from build123d import *

# Parameters (mm, degrees)
MAIN_DEPTH                   = 37.5
SKETCH2_W                    = 41
SKETCH2_H                    = 21
SERVOPLACE_DEPTH             = 11
SKETCH3_R                    = 1.25
SERVOFIXHOLE_DEPTH           = 11
SKETCH4_W                    = 10
SKETCH4_H                    = 10
CUTFORFIXMAKERBEAMHOLE_DEPTH = 18
SKETCH5_R                    = 1.5
FIXHOLEMAKERBEAM_DEPTH       = 9
FILLET1_R                    = 1


with BuildPart() as part:
    # Sketch1 → Main (new body, symmetric)
    with BuildSketch(Plane.XY):
        Polygon((-5, 0), (-5, 25), (5, 25), (5, 0), (1.45, 0), (1.45, -1), (-1.45, -1), (-1.45, 0), align=None)
    extrude(amount=MAIN_DEPTH, both=True)

    # Sketch2 → ServoPlace (cut, through all)
    with BuildSketch(Plane.ZY.offset(5)):
        with Locations((0, 9.5)):
            Rectangle(SKETCH2_W, SKETCH2_H)
    extrude(amount=-SERVOPLACE_DEPTH, mode=Mode.SUBTRACT)

    # Sketch3 → ServoFixHole (cut, through all)
    with BuildSketch(Plane.ZY.offset(5)):
        with Locations((-24.5, 15)):
            Circle(SKETCH3_R)
        with Locations((-24.5, 5)):
            Circle(SKETCH3_R)
    servofixhole = extrude(amount=-SERVOFIXHOLE_DEPTH, mode=Mode.SUBTRACT)

    # ServoFixHoleMirror: ServoFixHole across plane
    add(servofixhole.mirror(Plane.XY), mode=Mode.SUBTRACT)

    # Sketch4 → CutForFixMakerBeamHole (cut)
    with BuildSketch(Plane(origin=(0, 25, 0), x_dir=(1, 0, 0), z_dir=(0, 1, 0))):
        with Locations((0, 32.5)):
            Rectangle(SKETCH4_W, SKETCH4_H)
        with Locations((0, -32.5)):
            Rectangle(SKETCH4_W, SKETCH4_H)
    extrude(amount=-CUTFORFIXMAKERBEAMHOLE_DEPTH, mode=Mode.SUBTRACT)

    # Sketch5 → FixHoleMakerBeam (cut, through all)
    with BuildSketch(Plane(origin=(0, 7, 0), x_dir=(1, 0, 0), z_dir=(0, 1, 0))):
        with Locations((0, 32.5)):
            Circle(SKETCH5_R)
        with Locations((0, -32.5)):
            Circle(SKETCH5_R)
    extrude(amount=-FIXHOLEMAKERBEAM_DEPTH, mode=Mode.SUBTRACT)

    # Fillet1
    fillet1_edges = [part.edges().sort_by_distance(p)[0] for p in [
        (0, 7, -27.5),
        (0, 7, 27.5),
    ]]
    fillet(fillet1_edges, radius=FILLET1_R)


solid = part.part
Can you work these out from the model? Positions are in its coordinate system, mm. A direction names the side the tool comes from. Round coordinates to 2 decimals unless told otherwise and drop trailing zeros. Order: outer loops, then holes, each group sorted by start corner. A loop starts at its lowest first (then second) coordinate and runs counter-clockwise, first axis right, second up. Notation, with made-up numbers: (66.5, 10.5) - (86.5, 10.5) arc R31 cw to (86.5, 36.5) - close; hole circle Ø8 at (52.25, 30). An arc over 180 degrees is marked (long way). Answer in a Markdown table with one row per item.
(1) Suppose I cut it at C-C, the plane z = -24.5. Please give me the cut outline in (x, y).
From the geometry:
| item | result |
|---|---|
| outline | (-5, 0) - (-1.45, 0) - (-1.45, -1) - (1.45, -1) - (1.45, 0) - (5, 0) - (5, 3.75) - (-5, 3.75) - close; (-5, 6.25) - (5, 6.25) - (5, 13.75) - (-5, 13.75) - close; (-5, 16.25) - (5, 16.25) - (5, 25) - (-5, 25) - close |
(2) Which directions (+Z, -Z, +X, -X, +Y, -Y) give clear straight access to the entire face, cutting with the end or side of a thin tool? Please do faces 1 (the face through (3, 0, -29)), 2 (the face through (0, 17, -27.5)), 3 (the face through (0, 9, 20.5)), 4 (the face through (-3, 0, 29)).
From the geometry:
| item | result |
|---|---|
| face 1 | +Z, -Z, +X, -Y |
| face 2 | -Z, +X, -X, +Y |
| face 3 | +X, -X, -Y |
| face 4 | +Z, -Z, -X, -Y |
(3) Suppose I cut it at D-D, the plane y = 1. Please give me the cut outline in (x, z).
From the geometry:
| item | result |
|---|---|
| outline | (-5, -37.5) - (5, -37.5) - (5, -20.5) - (-5, -20.5) - close; (-5, 20.5) - (5, 20.5) - (5, 37.5) - (-5, 37.5) - close; hole circle Ø3 at (0, -32.5); hole circle Ø3 at (0, 32.5) |
(4) Please list where these lines run through material, in increasing order: L1, parallel to Y at x = -1.75, z = -24.5; L2, parallel to Z at x = 0, y = 1; L3, parallel to X at y = 1, z = 32.5. Write a range as from..to.
From the geometry:
| item | result |
|---|---|
| L1 | y = 0..3.75, 6.25..13.75, 16.25..25 |
| L2 | z = -37.5..-34, -31..-20.5, 20.5..31, 34..37.5 |
| L3 | x = -5..-1.5, 1.5..5 |
(5) If we mould it in two halves opening along Y, with no side actions, what happens to faces 5 (the face through (-0.07, 4.521, 23.345)), 6 (the face through (0, -1, -26)), 7 (the face through (0, 3, 37.5))? For each: released by +Y, released by -Y, zero draft, split by the parting line, or undercut.
From the geometry:
| item | result |
|---|---|
| face 5 | undercut |
| face 6 | released by -Y |
| face 7 | zero draft |
(6) For P1, Ø1.8, axis at x = -3.5, z = -32, coming from the -Y side; P2, Ø8, axis at y = 13, z = 4, coming from the -X side; P3, Ø2, axis at x = -2.5, z = -5.5, coming from the -Y side; P4, Ø3, axis at x = 1, y = 13, coming from the -Z side, each with a flat end and sliding along its axis, tell me the tip position at first contact or that it passes through.
From the geometry:
| item | result |
|---|---|
| P1 | stops at y = 0 |
| P2 | passes through |
| P3 | stops at y = 20 |
| P4 | stops at z = -27.5 |
(7) Suppose I cut it at B-B, the plane x = 0. Please give me the cut outline in (y, z), plus the area to 3 significant figures.
From the geometry:
| item | result |
|---|---|
| outline | (-1, -37.5) - (7, -37.5) - (7, -34) - (-1, -34) - close; (-1, -31) - (7, -31) - (7, -28.5) arc R1 cw to (8, -27.5) - (25, -27.5) - (25, 27.5) - (8, 27.5) arc R1 cw to (7, 28.5) - (7, 31) - (-1, 31) - (-1, 20.5) - (20, 20.5) - (20, -20.5) - (-1, -20.5) - close; (-1, 34) - (7, 34) - (7, 37.5) - (-1, 37.5) - close; hole circle Ø2.5 at (5, -24.5); hole circle Ø2.5 at (5, 24.5); hole circle Ø2.5 at (15, -24.5); hole circle Ø2.5 at (15, 24.5) |
| area | 662 mm2 |
(8) Suppose I cut it at A-A, the plane y = 5. Please give me the cut outline in (x, z), plus the area to 3 significant figures.
From the geometry:
| item | result |
|---|---|
| outline | (-5, -37.5) - (5, -37.5) - (5, -25.75) - (-5, -25.75) - close; (-5, -23.25) - (5, -23.25) - (5, -20.5) - (-5, -20.5) - close; (-5, 20.5) - (5, 20.5) - (5, 23.25) - (-5, 23.25) - close; (-5, 25.75) - (5, 25.75) - (5, 37.5) - (-5, 37.5) - close; hole circle Ø3 at (0, -32.5); hole circle Ø3 at (0, 32.5) |
| area | 276 mm2 |
